CAD build for the part. Positions are in the model's coordinates, mm. Face numbers are marked on the shaded views. A direction names the side the tool comes from. Round coordinates to 2 decimals unless told otherwise and drop trailing zeros. Write each loop counter-clockwise with the first axis right and the second up, starting at its lowest first coordinate (ties: lowest second). Pieces come first, ordered by that corner, then holes. Notation, with made-up numbers: (59.25, 9.5) - (115.25, 9.5) arc R21 ccw to (115.25, 44.5) - close; hole circle Ø11 at (70, 46.25). An arc over 180 degrees is marked (long way). Use one line per item in the form item = value. Start each with the question number.
Item 1: Band-saw the part on D-D, the plane z = 20. List the corners of the cut face in (x, y).
Item 2: Pin check, flat tips, straight feed: pin 1 (1.6 mm diameter, centred on x = -44, z = 8, fed in from -Y); pin 2 (5.5 mm diameter, centred on x = 69, z = 51.5, fed in from -Y); pin 3 (9 mm diameter, centred on x = -45.5, y = -2, fed in from +Z). Stop position of each tip, or through.
Item 3: Band-saw the part on A-A, the plane z = 50. List the corners of the cut face in (x, y), and give its area (3 significant figures).
Item 4: Tool access for the marked faces 1, 2, 3 and 4: list every direction of +Z, -Z, +X, -X, +Y, -Y with a clear straight run to the whole face (end or side of a thin tool).
Item 5: Band-saw the part on C-C, the plane y = 25.5. List the corners of the cut face in (x, z).
Item 6: Drill centre lines: L1, parallel to Z at x = -49.5, y = 0; L2, parallel to Y at x = -38.75, z = 0; L3, parallel to Z at x = 24, y = -58. Where is each one in solid material? Low to high.
Item 7: Band-saw the part on B-B, the plane x = 126. List the corners of the cut face in (y, z).
from build123d import *

# Parameters (mm, degrees)
SKETCH1_W                       = 130
SKETCH1_H                       = 130
BOSS_EXTRUDE1_DEPTH             = 11.5
FILLET1_R                       = 10
BOSS_EXTRUDE2_DEPTH             = 204.5
SKETCH3_R                       = 55
BOSS_EXTRUDE3_DEPTH             = 6
SKETCH4_R                       = 11
BOSS_EXTRUDE4_DEPTH             = 55
CUT_EXTRUDE1_START              = 7
CUT_EXTRUDE1_DEPTH              = 113
M6X1_0_TAPPED_HOLE1_D           = 5
M6X1_0_TAPPED_HOLE1_DEPTH       = 20
M6X1_0_TAPPED_HOLE1_CSINK_D     = 6.05
M6X1_0_TAPPED_HOLE1_CSINK_ANGLE = 90
M6X1_0_TAPPED_HOLE1_TIP         = 1.502151548
SKETCH9_R                       = 4.5
CUT_EXTRUDE2_DEPTH              = 20
FILLET2_R                       = 3


with BuildPart() as part:
    # Sketch1 → Boss-Extrude1 (new body)
    with BuildSketch(Plane(origin=(0, 0, 0), x_dir=(0, 0, -1), z_dir=(1, 0, 0))):
        Rectangle(SKETCH1_W, SKETCH1_H)
    extrude(amount=BOSS_EXTRUDE1_DEPTH)

    # Fillet1
    fillet1_edges = [part.edges().sort_by_distance(p)[0] for p in [
        (5.75, -65, -65),
        (5.75, -65, 65),
        (5.75, 65, 65),
        (5.75, 65, -65),
    ]]
    fillet(fillet1_edges, radius=FILLET1_R)

    # Sketch2 → Boss-Extrude2 (add)
    with BuildSketch(Plane(origin=(11.5, 0, 0), x_dir=(0, 0, -1), z_dir=(1, 0, 0))):
        Polygon((-40, 65), (40, 65), (40, 40), (65, 40), (65, -40), (40, -40), (40, -65), (-40, -65), (-40, -40), (-65, -40), (-65, 40), (-40, 40), align=None)
    extrude(amount=BOSS_EXTRUDE2_DEPTH)

    # Sketch3 → Boss-Extrude3 (add)
    with BuildSketch(Plane.ZY):
        Circle(SKETCH3_R)
    extrude(amount=BOSS_EXTRUDE3_DEPTH)

    # Sketch4 → Boss-Extrude4 (add)
    with BuildSketch(Plane.ZY):
        Circle(SKETCH4_R)
    extrude(amount=BOSS_EXTRUDE4_DEPTH)

    # Sketch6 → Cut-Extrude1 (cut)
    with BuildSketch(Plane.XY.offset(CUT_EXTRUDE1_START)):
        with BuildLine():
            Line((-55, 4), (-23, 4))
            ThreePointArc((-23, 4), (-19, 0), (-23, -4))
            Line((-23, -4), (-55, -4))
            ThreePointArc((-55, -4), (-59, 0), (-55, 4))
        make_face()
    extrude(amount=CUT_EXTRUDE1_DEPTH, mode=Mode.SUBTRACT)

    # M6x1.0 Tapped Hole1
    with Locations(Plane.ZY.offset(55)):
        with Locations((0, 0)):
            CounterSinkHole(M6X1_0_TAPPED_HOLE1_D / 2, M6X1_0_TAPPED_HOLE1_CSINK_D / 2, depth=M6X1_0_TAPPED_HOLE1_DEPTH, counter_sink_angle=M6X1_0_TAPPED_HOLE1_CSINK_ANGLE)
            with Locations((0, 0, -(M6X1_0_TAPPED_HOLE1_DEPTH + M6X1_0_TAPPED_HOLE1_TIP / 2))):  # 118° drill point
                Cone(0, M6X1_0_TAPPED_HOLE1_D / 2, M6X1_0_TAPPED_HOLE1_TIP, mode=Mode.SUBTRACT)

    # Sketch9 → Cut-Extrude2 (cut)
    with BuildSketch(Plane.ZY):
        with Locations((51.265241636, 51.265241636)):
            Circle(SKETCH9_R)
        with Locations((51.265241636, -51.265241636)):
            Circle(SKETCH9_R)
        with Locations((-51.265241636, -51.265241636)):
            Circle(SKETCH9_R)
        with Locations((-51.265241636, 51.265241636)):
            Circle(SKETCH9_R)
    extrude(amount=-CUT_EXTRUDE2_DEPTH, mode=Mode.SUBTRACT)

    # Fillet2
    fillet2_edges = [part.edges().sort_by_distance(p)[0] for p in [
        (113.75, 65, 40),
        (113.75, 40, 40),
        (113.75, 40, 65),
        (113.75, -40, 65),
        (113.75, -40, 40),
        (113.75, -65, 40),
        (113.75, -65, -40),
        (113.75, -40, -40),
        (113.75, -40, -65),
        (113.75, 40, -65),
        (113.75, 40, -40),
        (113.75, 65, -40),
        (216, 52.5, 40),
        (216, 40, 52.5),
        (216, 0, 65),
        (216, -40, 52.5),
        (216, -52.5, 40),
        (216, -65, 0),
        (216, -52.5, -40),
        (216, -40, -52.5),
        (216, 0, -65),
        (216, 40, -52.5),
        (216, 52.5, -40),
        (216, 65, 0),
    ]]
    fillet(fillet2_edges, radius=FILLET2_R)


solid = part.part
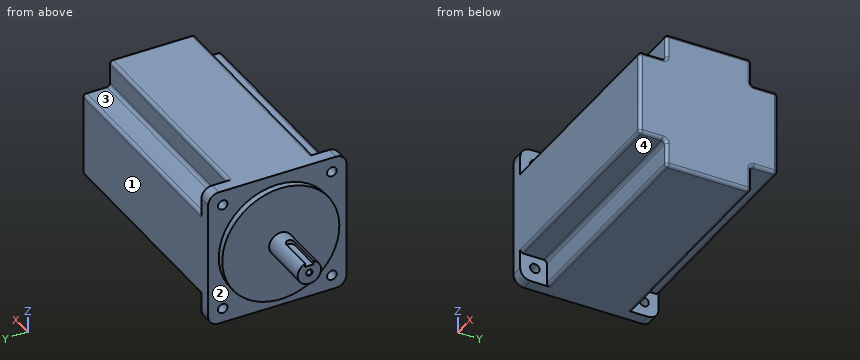
Determined:
q1.outline = (-6, -51.23) - (0, -51.23) - (0, -65) - (213, -65) arc R3 ccw to (216, -62) - (216, 62) arc R3 ccw to (213, 65) - (0, 65) - (0, 51.23) - (-6, 51.23) - close
q2.pin_1 = -8.32
q2.pin_2 = -40
q2.pin_3 = 10.25
q3.outline = (-6, -22.91) - (0, -22.91) - (0, -46.95) - (11.5, -46.95) - (11.5, -40) - (213, -40) arc R3 ccw to (216, -37) - (216, 37) arc R3 ccw to (213, 40) - (11.5, 40) - (11.5, 46.95) - (0, 46.95) - (0, 22.91) - (-6, 22.91) - close; (0, -65) - (11.5, -65) - (11.5, -55.58) - (0, -55.58) - close; (0, 55.58) - (11.5, 55.58) - (11.5, 65) - (0, 65) - close
q3.area = 17,900 mm²
q4.face_1 = +Z, -Z, +X, -X, +Y
q4.face_2 = -X
q4.face_3 = +Z, +X, +Y
q4.face_4 = -Z, +X, -Y
q5.outline = (-6, -48.73) - (0, -48.73) - (0, -65) - (213, -65) arc R3 ccw to (216, -62) - (216, 62) arc R3 ccw to (213, 65) - (0, 65) - (0, 48.73) - (-6, 48.73) - close
q6.L1 = -11 to -2.5, 2.5 to 7
q6.L2 = -11 to -2.5, 2.5 to 11
q6.L3 = -40 to 40
q7.outline = (-65, -37) arc R3 ccw to (-62, -40) - (-43, -40) arc R3 cw to (-40, -43) - (-40, -62) arc R3 ccw to (-37, -65) - (37, -65) arc R3 ccw to (40, -62) - (40, -43) arc R3 cw to (43, -40) - (62, -40) arc R3 ccw to (65, -37) - (65, 37) arc R3 ccw to (62, 40) - (43, 40) arc R3 cw to (40, 43) - (40, 62) arc R3 ccw to (37, 65) - (-37, 65) arc R3 ccw to (-40, 62) - (-40, 43) arc R3 cw to (-43, 40) - (-62, 40) arc R3 ccw to (-65, 37) - close
